Geometry check sheet. Reference: the model listing, model coordinates, mm. A direction names the side the tool comes from. Round coordinates to 2 decimals unless told otherwise and drop trailing zeros. Write each loop counter-clockwise with the first axis right and the second up, starting at its lowest first coordinate (ties: lowest second). Pieces come first, ordered by that corner, then holes.
Item 1: Depth check by flat-ended pin: P1, Ø5, axis at x = -49.52, z = -24.88, coming from the +Y side; P2, Ø1.5, axis at x = -29.5, y = -1, coming from the +Z side. Enter the tip coordinate at first touch or a pass-through.
Item 2: Cross-section at C-C (z = 88). Enter the section's corners in (x, y), then the cut area to 3 significant figures.
Item 3: Cross-section at B-B (x = -54.5). Enter the section's corners in (y, z), then the cut area to 3 significant figures.
Item 4: Scan lines: probe 1 along Z at (x, y) = (-50, -1.65); probe 2 along Z at (x, y) = (-48, -0.05); probe 3 along Z at (x, y) = (-53.5, -0.6). Record each from-to range of solid material in increasing order.
Item 5: Cross-section at D-D (x = -14). Enter the section's corners in (y, z), then the cut area to 3 significant figures.
Item 6: Draft check along Z on faces 1 (the face through (-47, -3.048, 34)), 2 (the face through (-18, -2, -16.943)), 3 (the face through (-49.76, -1.5, 73.93)), 4 (the face through (-37.403, -1.503, -14.322)). Enter one of: pulls with the +Z half, pulls with the -Z half, needs draft (parallel to the pull), parting line crosses it, or undercut.
Item 7: Cross-section at A-A (y = -1.25). State how many separate pieces and enclosed holes the cut face has, then the cut area to 3 significant figures.
Item 8: Access from +Z, -Z, +X, -X, +Y, -Y to the whole of each face (thin tool, end or side, straight path). Record for faces 5 (the face through (-28, -2, -32.818)), 6 (the face through (-36.618, -1.503, 14.005)).
from build123d import *

# Parameters (mm, degrees)
F0_R     = 3.175
F1_DEPTH = 3.048


with BuildPart() as f1:
    # F0 (on Front) → F1 (new body)
    with BuildSketch(Plane.XZ):
        with BuildLine():
            ThreePointArc((-58.9681591883, 90.6098637193), (-56.6616162241, 83.1190434099), (-49.5178662241, 79.8942387193))
            ThreePointArc((-49.5178662241, 79.8942387193), (-42.7826741332, 82.6840466285), (-39.9928662241, 89.4192387193))
            ThreePointArc((-39.9928662241, 89.4192387193), (-40.0115613298, 90.0157219613), (-40.0675732598, 90.6098637193))
            ThreePointArc((-40.0675732598, 90.6098637193), (-49.5178662241, 98.9442387193), (-58.9681591883, 90.6098637193))
        make_face()
        with BuildLine():
            ThreePointArc((-46.3428662241, 89.4192387193), (-47.2728021938, 87.1741746891), (-49.5178662241, 86.2442387193))
            ThreePointArc((-49.5178662241, 86.2442387193), (-51.7629302543, 91.6643027496), (-46.3428662241, 89.4192387193))
        make_face(mode=Mode.SUBTRACT)
        with BuildLine():
            ThreePointArc((-39.9928662241, 89.4192387193), (-42.7826741332, 82.6840466285), (-49.5178662241, 79.8942387193))
            Line((-49.5178662241, 79.8942387193), (-49.5178662241, 75.1444387193))
            Line((-49.5178662241, 75.1444387193), (-49.5178662241, 54.4942387193))
            ThreePointArc((-49.5178662241, 54.4942387193), (-39.0175407083, 50.5254887193), (-33.7673779504, 40.6036137193))
            Line((-33.7673779504, 40.6036137193), (-40.0675732598, 90.6098637193))
            ThreePointArc((-40.0675732598, 90.6098637193), (-40.0115613298, 90.0157219613), (-39.9928662241, 89.4192387193))
        make_face()
        with BuildLine():
            Line((-49.5178662241, 75.1444387193), (-49.5178662241, 79.8942387193))
            ThreePointArc((-49.5178662241, 79.8942387193), (-56.6616162241, 83.1190434099), (-58.9681591883, 90.6098637193))
            Line((-58.9681591883, 90.6098637193), (-65.2683544977, 40.6036137193))
            ThreePointArc((-65.2683544977, 40.6036137193), (-60.0181917398, 50.5254887193), (-49.5178662241, 54.4942387193))
            Line((-49.5178662241, 54.4942387193), (-49.5178662241, 75.1444387193))
        make_face()
        with Locations((-52.6928662241, 75.1444387193)):
            Circle(F0_R, mode=Mode.SUBTRACT)
        with BuildLine():
            ThreePointArc((-33.7673779504, 40.6036137193), (-39.0175407083, 50.5254887193), (-49.5178662241, 54.4942387193))
            Line((-49.5178662241, 54.4942387193), (-49.5178662241, 42.1952313846))
            ThreePointArc((-49.5178662241, 42.1952313846), (-46.9892575609, 41.1478473825), (-45.9418735588, 38.6192387193))
            ThreePointArc((-45.9418735588, 38.6192387193), (-46.9892575609, 36.0906300562), (-49.5178662241, 35.043246054))
            Line((-49.5178662241, 35.043246054), (-49.5178662241, 22.7442387193))
            ThreePointArc((-49.5178662241, 22.7442387193), (-39.0175407083, 26.7129887193), (-33.7673779504, 36.6348637193))
            ThreePointArc((-33.7673779504, 36.6348637193), (-33.6740247337, 37.6250999827), (-33.6428662241, 38.6192387193))
            ThreePointArc((-33.6428662241, 38.6192387193), (-33.6740247337, 39.613377456), (-33.7673779504, 40.6036137193))
        make_face()
        with BuildLine():
            Line((-49.5178662241, 42.1952313846), (-49.5178662241, 54.4942387193))
            ThreePointArc((-49.5178662241, 54.4942387193), (-60.0181917398, 50.5254887193), (-65.2683544977, 40.6036137193))
            ThreePointArc((-65.2683544977, 40.6036137193), (-65.3928662241, 38.6192387193), (-65.2683544977, 36.6348637193))
            ThreePointArc((-65.2683544977, 36.6348637193), (-60.0181917398, 26.7129887193), (-49.5178662241, 22.7442387193))
            Line((-49.5178662241, 22.7442387193), (-49.5178662241, 35.043246054))
            ThreePointArc((-49.5178662241, 35.043246054), (-53.0938588894, 38.6192387193), (-49.5178662241, 42.1952313846))
        make_face()
        with BuildLine():
            ThreePointArc((-49.5178662241, 22.7442387193), (-60.0181917398, 26.7129887193), (-65.2683544977, 36.6348637193))
            Line((-65.2683544977, 36.6348637193), (-57.3931103609, -25.8729487807))
            ThreePointArc((-57.3931103609, -25.8729487807), (-55.4709912241, -19.6305985228), (-49.5178662241, -16.9432612807))
            Line((-49.5178662241, -16.9432612807), (-49.5178662241, 22.7442387193))
        make_face()
        with BuildLine():
            ThreePointArc((-33.7673779504, 36.6348637193), (-39.0175407083, 26.7129887193), (-49.5178662241, 22.7442387193))
            Line((-49.5178662241, 22.7442387193), (-49.5178662241, -16.9432612807))
            ThreePointArc((-49.5178662241, -16.9432612807), (-43.9052061484, -19.268101205), (-41.5803662241, -24.8807612807))
            Line((-41.5803662241, -24.8807612807), (-13.0053662241, -24.8807612807))
            ThreePointArc((-13.0053662241, -24.8807612807), (-10.6805262997, -19.268101205), (-5.0678662241, -16.9432612807))
            Line((-5.0678662241, -16.9432612807), (-31.5029077506, -16.9432612807))
            ThreePointArc((-31.5029077506, -16.9432612807), (-37.4655577506, -14.251624299), (-39.390752278, -7.9992862807))
            Line((-39.390752278, -7.9992862807), (-33.7673779504, 36.6348637193))
        make_face()
        with BuildLine():
            ThreePointArc((-49.5178662241, -16.9432612807), (-55.4709912241, -19.6305985228), (-57.3931103609, -25.8729487807))
            ThreePointArc((-57.3931103609, -25.8729487807), (-54.7680289819, -30.8338862807), (-49.5178662241, -32.8182612807))
            ThreePointArc((-49.5178662241, -32.8182612807), (-43.9052061484, -30.4934213563), (-41.5803662241, -24.8807612807))
            Line((-41.5803662241, -24.8807612807), (-46.3166417574, -24.8807612807))
            ThreePointArc((-46.3166417574, -24.8807612807), (-51.7814737525, -27.1443688092), (-49.5178662241, -21.679536814))
            Line((-49.5178662241, -21.679536814), (-49.5178662241, -16.9432612807))
        make_face()
        with BuildLine():
            ThreePointArc((-41.5803662241, -24.8807612807), (-43.9052061484, -30.4934213563), (-49.5178662241, -32.8182612807))
            Line((-49.5178662241, -32.8182612807), (-5.0678662241, -32.8182612807))
            ThreePointArc((-5.0678662241, -32.8182612807), (-10.6805262997, -30.4934213563), (-13.0053662241, -24.8807612807))
            Line((-13.0053662241, -24.8807612807), (-41.5803662241, -24.8807612807))
        make_face()
        with BuildLine():
            ThreePointArc((-13.0053662241, -24.8807612807), (-10.6805262997, -30.4934213563), (-5.0678662241, -32.8182612807))
            ThreePointArc((-5.0678662241, -32.8182612807), (0.5447938516, -30.4934213563), (2.8696337759, -24.8807612807))
            ThreePointArc((2.8696337759, -24.8807612807), (0.5447938516, -19.268101205), (-5.0678662241, -16.9432612807))
            ThreePointArc((-5.0678662241, -16.9432612807), (-10.6805262997, -19.268101205), (-13.0053662241, -24.8807612807))
        make_face()
        with BuildLine():
            ThreePointArc((-41.5803662241, -24.8807612807), (-43.9052061484, -19.268101205), (-49.5178662241, -16.9432612807))
            Line((-49.5178662241, -16.9432612807), (-49.5178662241, -21.679536814))
            ThreePointArc((-49.5178662241, -21.679536814), (-47.2542586956, -22.6171537522), (-46.3166417574, -24.8807612807))
            Line((-46.3166417574, -24.8807612807), (-41.5803662241, -24.8807612807))
        make_face()
    extrude(amount=F1_DEPTH)


solid = f1.part
Resolved:
1. P1: passes through
1. P2: stops at z = -16.94
2. outline: (-59.3, -3.05) - (-52.36, -3.05) - (-52.36, 0) - (-59.3, 0) - close; (-46.68, -3.05) - (-39.74, -3.05) - (-39.74, 0) - (-46.68, 0) - close
2. area: 42.3 mm2
3. outline: (-3.05, -31.06) - (0, -31.06) - (0, 72.53) - (-3.05, 72.53) - close; (-3.05, 77.75) - (0, 77.75) - (0, 97.54) - (-3.05, 97.54) - close
3. area: 376 mm2
4. probe 1: z = -32.8 to -28.05, -21.72 to 35.08, 42.16 to 73.46, 76.83 to 86.28, 92.56 to 98.93
4. probe 2: z = -32.82 to -27.7, -22.06 to 35.38, 41.86 to 86.63, 92.21 to 98.82
4. probe 3: z = -31.75 to 72.07, 78.22 to 98.07
5. outline: (-3.05, -32.82) - (0, -32.82) - (0, -16.94) - (-3.05, -16.94) - close
5. area: 48.4 mm2
6. face 1: needs draft
6. face 2: pulls with the +Z half
6. face 3: undercut
6. face 4: undercut
7. separate pieces: 1
7. enclosed holes: 4
7. area: 3,640 mm2
8. face 5: -Z, +X, -X, +Y, -Y
8. face 6: +X, +Y, -Y
